```python
from build123d import *

# Parameters (mm, degrees)
BOSS_EXTRUDE1_DEPTH = 4
BOSS_EXTRUDE1_DRAFT = 1
SHELL1_T            = -0.5
SKETCH2_R           = 2
BOSS_EXTRUDE2_DEPTH = 5.5
BOSS_EXTRUDE2_TAPER = 1.5
RIB1_START          = -0.25
RIB1_DEPTH          = 0.5
CIRPATTERN1_COUNT   = 4


# Read off the part's stored shape, not the designer's step: Rib1
with BuildPart() as part:
    # Sketch1 → Boss-Extrude1 (with draft: the straight prism first)
    with BuildSketch(Plane(origin=(0, 0, 0), x_dir=(1, 0, 0), z_dir=(0, 1, 0))):
        with BuildLine():
            Line((-7.5, -6.375), (7.5, -6.375))
            ThreePointArc((7.5, -6.375), (8.207106781, -6.082106781), (8.5, -5.375))
            Line((8.5, -5.375), (8.5, 5.375))
            ThreePointArc((8.5, 5.375), (8.207106781, 6.082106781), (7.5, 6.375))
            Line((7.5, 6.375), (-7.5, 6.375))
            ThreePointArc((-7.5, 6.375), (-8.207106781, 6.082106781), (-8.5, 5.375))
            Line((-8.5, 5.375), (-8.5, -5.375))
            ThreePointArc((-8.5, -5.375), (-8.207106781, -6.082106781), (-7.5, -6.375))
        make_face()
    extrude(amount=-BOSS_EXTRUDE1_DEPTH)
    # Boss-Extrude1: the draft: its side faces are tilted about the plane it starts from
    boss_extrude1_sides = [part.faces().sort_by_distance(p)[0] for p in [
        (0, -2, 6.375),
        (8.207106781, -2, 6.082106781),
        (8.5, -2, 0),
        (8.207106781, -2, -6.082106781),
        (0, -2, -6.375),
        (-8.207106781, -2, -6.082106781),
        (-8.5, -2, 0),
        (-8.207106781, -2, 6.082106781),
    ]]
    draft(boss_extrude1_sides, Plane(origin=(0, 0, 0), x_dir=(1, 0, 0), z_dir=(0, 1, 0)), BOSS_EXTRUDE1_DRAFT)

    # Shell1
    shell1_openings = [part.faces().sort_by_distance(p)[0] for p in [
        (0, -4, 0),
    ]]
    offset(amount=SHELL1_T, openings=shell1_openings, kind=Kind.INTERSECTION)

    # Sketch2 → Boss-Extrude2 (add)
    with BuildSketch(Plane.XZ.offset(0.5)):
        Circle(SKETCH2_R)
    extrude(amount=BOSS_EXTRUDE2_DEPTH, taper=BOSS_EXTRUDE2_TAPER)

    # Rib1 outline → Rib1 (add)
    with BuildSketch(Plane.XY.offset(RIB1_START)):
        Polygon((-2.392140648, -4.618982479), (-1, -4.618982479), (-1, 0), (-3.073787562, 0), (-3, -0.5), align=None)
    rib1 = extrude(amount=RIB1_DEPTH)

    # CirPattern1: Rib1 ×4 about axis
    cirpattern1_axis = Axis((0, 0, 0), (0, 1, 0))
    for i in range(1, CIRPATTERN1_COUNT):
        add(rib1.rotate(cirpattern1_axis, i * 360 / CIRPATTERN1_COUNT))


solid = part.part
```
Read the model definition and answer for the solid it produces. Units are mm, in the model's axes. A direction names the side the tool comes from. Round coordinates to 2 decimals unless told otherwise and drop trailing zeros. Write each loop counter-clockwise with the first axis right and the second up, starting at its lowest first coordinate (ties: lowest second). Pieces come first, ordered by that corner, then holes. Notation, with made-up numbers: M -22,78 L -16,78 A22 ccw -16,108 Z; hole C 30.25,2 d9. An arc over 180 degrees is marked long. One line per item, written item: value.
Q1. Flat-ended cylindrical pins translate along their axes: pin 1 Ø1.2 at (y, z) = (-2.5, 2.5) entering from +X; pin 2 Ø0.9 at (x, y) = (-2.5, -2.5) entering from -Z; pin 3 Ø0.6 at (y, z) = (-2.5, -2.5) entering from +X. Find the tip coordinate at first contact, or state that the pin passes through.
Data:
pin 1: x = 8.55
pin 2: z = -6.43
pin 3: x = 8.55
Q2. Straight lines are drawn through the part: line 1 (Z direction, x = 1.5, y = -2.75); line 2 (X direction, y = -3.75, z = 4); line 3 (X direction, y = -2.5, z = -2.25). For each, find the intervals that lie inside material, in ascending order. Write a range as [from, to].
Data:
line 1: [-6.42, -5.92], [-1.23, 1.23], [5.92, 6.42]
line 2: [-8.57, -8.07], [8.07, 8.57]
line 3: [-8.54, -8.04], [-0.25, 0.25], [8.04, 8.54]
Q3. Which of the six approach directions +Z, -Z, +X, -X, +Y, -Y give full straight-line access (tool end or side, diameter ignored) to faces 4 (the flat face through (0.25, -2.5, 2.3)), 5 (the conical face through (8.223, -1.972, 6.114)), 6 (the flat face through (0, -6, 0))?
Data:
face 4: -Y
face 5: +Z, +X, +Y
face 6: +Z, -Z, +X, -X, -Y
Q4. Find section C-C on x = -6.5. Write down the section's boundary in (y, z) (3 decimals), plus the area to 3 significant figures.
Data:
outline: M -4,-6.445 L 0,-6.375 L 0,6.375 L -4,6.445 L -4,5.945 L -0.5,5.884 L -0.5,-5.884 L -4,-5.945 Z
area: 9.88 mm2
Q5. For a pull along Z with two mould halves and no side action, classify faces 1 (the conical face through (-8.24, -1.97, 6.1)), 2 (the flat face through (0.25, -2.5, -2.3)), 3 (the conical face through (8.24, -1.97, -6.1)) as +Z half, -Z half, draft (parallel to the pull), parting line (faces both ways), or undercut.
Data:
face 1: +Z half
face 2: undercut
face 3: -Z half
Q6. Find section A-A on y = -1.75. Count the separate pieces of the cut face and the enclosed holes in it, plus the area to 3 significant figures.
Data:
separate pieces: 2
enclosed holes: 1
area: 42.1 mm2
Q7. Find section B-B on z = 3.25. Write down the section's boundary in (x, y), plus the area to 3 significant figures.
Data:
outline: M -8.57,-4 L -8.07,-4 L -8.01,-0.5 L 8.01,-0.5 L 8.07,-4 L 8.57,-4 L 8.5,0 L -8.5,0 Z
area: 12.0 mm2
